Design review of the part shown in the three views and the two pictorial views. Dimensions are in mm from the part's minimum x, y and z. A direction names the side the tool comes from. Coordinates: 2 decimals unless noted, no trailing zeros. Loops run counter-clockwise (first coordinate to the right, second up) from the corner with the lowest first, then second, coordinate; pieces in that order, holes last. Notation, with made-up numbers: (-21, 26) -> (14, 26) arc R20 cw to (14, 32) -> close; hole circle Ø6 at (-24.75, 59.25). An arc over 180 degrees is marked (long way). Use a Markdown table: item, result. Add a question column.
Q1. For probe 1 along Y at (x, z) = (3.5, 1.9); probe 2 along X at (y, z) = (8.5, 0.65); probe 3 along X at (y, z) = (11, 3.75), list the stretches that pass through material, from the lowest coordinate up.
Q2. Take a section at A-A on z = 0.6. Write out the cut boundary in (x, y).
Q3. Clearance check with flat-ended pins moving along their axes: pin 1 Ø0.8 at (x, z) = (20.5, 0.5) entering from -Y; pin 2 Ø1.5 at (x, y) = (8, 9.5) entering from -Z; pin 3 Ø0.5 at (y, z) = (7.5, 0.5) entering from +X; pin 4 Ø2 at (x, z) = (24, 3) entering from -Y. State where each tip first meets the part, or that it passes through.
Q4. Take a section at C-C on x = 14.5. Write out the cut boundary in (y, z).
Q5. Take a section at D-D on y = 1.5. Write out the cut boundary in (x, z).
Q6. For the marked faces 1 and 2, list the 3-axis set-ups (+Z, -Z, +X, -X, +Y, -Y) from which the entire face can be reached by the end or side of a thin tool; tool diameter is ignored.
Q7. Take a section at B-B on y = 6. Write out the cut boundary in (x, z), plus the area to 3 significant figures.
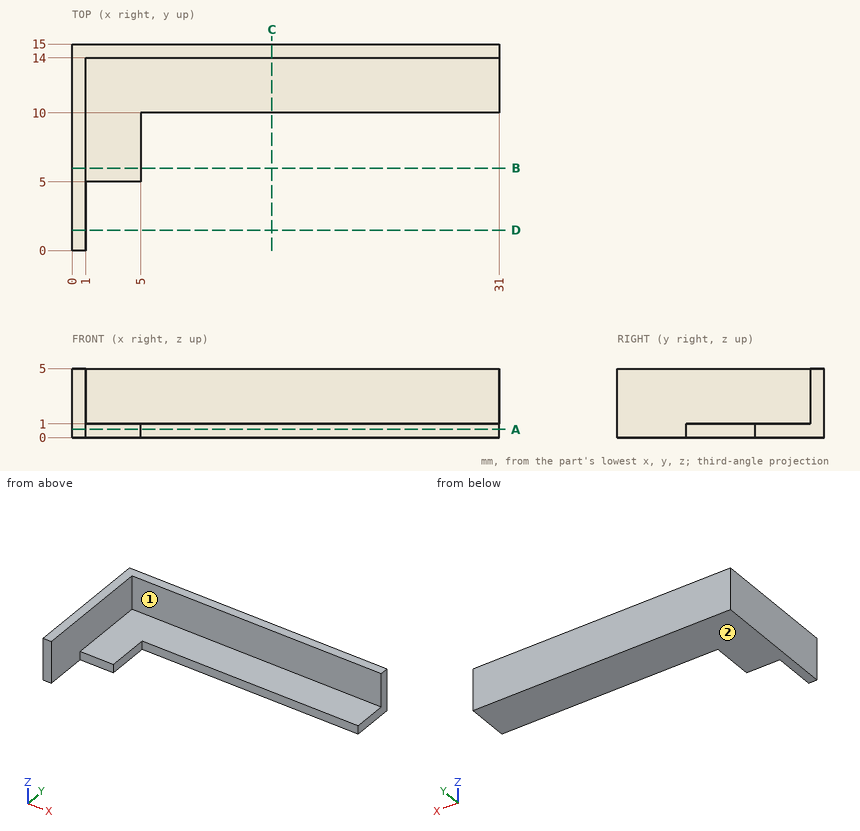
Answer list:
| question | item | result |
|---|---|---|
| 1 | probe 1 | 14 to 15 |
| 1 | probe 2 | 0 to 5 |
| 1 | probe 3 | 0 to 1 |
| 2 | outline | (0, 0) -> (1, 0) -> (1, 5) -> (5, 5) -> (5, 10) -> (31, 10) -> (31, 15) -> (0, 15) -> close |
| 3 | pin 1 | y = 10 |
| 3 | pin 2 | z = 0 |
| 3 | pin 3 | x = 5 |
| 3 | pin 4 | y = 14 |
| 4 | outline | (10, 0) -> (15, 0) -> (15, 5) -> (14, 5) -> (14, 1) -> (10, 1) -> close |
| 5 | outline | (0, 0) -> (1, 0) -> (1, 5) -> (0, 5) -> close |
| 6 | face 1 | +Z, +X, -Y |
| 6 | face 2 | -Z, +X, -X, +Y, -Y |
| 7 | outline | (0, 0) -> (5, 0) -> (5, 1) -> (1, 1) -> (1, 5) -> (0, 5) -> close |
| 7 | area | 9.00 mm² |
